Build history of the part. All positions in model axes, mm. A direction names the side the tool comes from. Coordinates: 2 decimals unless noted, no trailing zeros. Order: outer loops, then holes, each group sorted by start corner. A loop starts at its lowest first (then second) coordinate and runs counter-clockwise, first axis right, second up. Notation, with made-up numbers: (50.25, -31) - (69.25, -31) arc R16 cw to (69.25, -13) - close; hole circle Ø2 at (0.5, -5.75). An arc over 180 degrees is marked (long way). Write each question's results on one line, items separated by ' | '.
from build123d import *

# Parameters (mm, degrees)
BOSS_EXTRUDE1_DEPTH = 30
BOSS_EXTRUDE2_DEPTH = 30
SKETCH5_W           = 20
SKETCH5_H           = 30
CUT_EXTRUDE1_DEPTH  = 71
SKETCH6_W           = 30
SKETCH6_H           = 10
CUT_EXTRUDE2_DEPTH  = 40
CUT_EXTRUDE3_DEPTH  = 71


with BuildPart() as part:
    # Sketch1 → Boss-Extrude1 (new body)
    with BuildSketch(Plane(origin=(0, 0, 0), x_dir=(1, 0, 0), z_dir=(0, 1, 0))):
        Polygon((0, 0), (90, 0), (90, -70), (60, -70), (60, -60), (50, -60), (10, -40), (10, -30), (0, -30), align=None)
    extrude(amount=BOSS_EXTRUDE1_DEPTH)

    # Sketch3 → Boss-Extrude2 (add)
    with BuildSketch(Plane(origin=(0, 30, 0), x_dir=(1, 0, 0), z_dir=(0, 1, 0))):
        Polygon((0, 0), (90, 0), (90, -70), (60, -70), (60, -30), (0, -30), align=None)
    extrude(amount=BOSS_EXTRUDE2_DEPTH)

    # Sketch5 → Cut-Extrude1 (cut, through all)
    with BuildSketch(Plane.XY.offset(70)):
        with Locations((80, 25)):
            Rectangle(SKETCH5_W, SKETCH5_H)
    extrude(amount=-CUT_EXTRUDE1_DEPTH, mode=Mode.SUBTRACT)

    # Sketch6 → Cut-Extrude2 (cut)
    with BuildSketch(Plane.XY.offset(70)):
        with Locations((75, 55)):
            Rectangle(SKETCH6_W, SKETCH6_H)
    extrude(amount=-CUT_EXTRUDE2_DEPTH, mode=Mode.SUBTRACT)

    # Sketch7 → Cut-Extrude3 (cut, through all)
    with BuildSketch(Plane(origin=(0, 0, 0), x_dir=(-1, 0, 0), z_dir=(0, 0, -1))):
        Polygon((-40, 60), (-40, 50), (-20, 40), (0, 40), (0, 60), align=None)
    extrude(amount=-CUT_EXTRUDE3_DEPTH, mode=Mode.SUBTRACT)


solid = part.part
1. Band-saw the part on A-A on x = 81. Give the cut face in (y, z).
Solved:
outline: (0, 0) - (10, 0) - (10, 70) - (0, 70) - close; (40, 0) - (60, 0) - (60, 30) - (50, 30) - (50, 70) - (40, 70) - close
2. Band-saw the part on D-D on x = 25.5. Give the cut face in (y, z), then the cut area to 4 significant figures.
Solved:
outline: (0, 0) - (42.75, 0) - (42.75, 30) - (30, 30) - (30, 47.75) - (0, 47.75) - close | area: 1,815 mm2
3. Probe line 1 (Y direction, x = 70.5, z = 34); line 2 (X direction, y = 17, z = 16.5); line 3 (Y direction, x = 75, z = 26). List the from-to ranges inside material, lowest first.
Solved:
line 1: y = 0 to 10, 40 to 50 | line 2: x = 0 to 70 | line 3: y = 0 to 10, 40 to 60
4. Band-saw the part on B-B on z = 50.5. Give the cut face in (x, y), then the cut area to 3 significant figures.
Solved:
outline: (31, 0) - (90, 0) - (90, 10) - (70, 10) - (70, 40) - (90, 40) - (90, 50) - (60, 50) - (60, 30) - (31, 30) - close | area: 1,770 mm2
5. Tool access for faces 1 (the face through (10, 40, 15)), 2 (the face through (41, 30, 41)), 3 (the face through (80, 40, 35)), 4 (the face through (75, 50, 50)), 5 (the face through (10, 15, 35)): list every direction of +Z, -Z, +X, -X, +Y, -Y with a clear straight run to the whole face (end or side of a thin tool).
Solved:
face 1: +Z, -Z, -X, +Y | face 2: +Z, -X, +Y | face 3: +Z, -Z, +X | face 4: +Z, +X, -X, +Y | face 5: +Z, -X, +Y, -Y
6. Two-plate mould, pull along Y, no slides. Class faces 6 (the face through (80, 10, 35)), 7 (the face through (65, 60, 15)), 8 (the face through (44, 30, 0)), 9 (the face through (56, 0, 27)): +Y half, -Y half, draft (parallel to the pull), parting line (faces both ways), or undercut.
Solved:
face 6: undercut | face 7: +Y half | face 8: draft | face 9: -Y half
7. Drop flat-ended pins along their axis: pin 1 Ø10 at (y, z) = (53.5, 19.5) entering from -X; pin 2 Ø1 at (x, y) = (50, 32) entering from +Z; pin 3 Ø11 at (y, z) = (56.5, 8.5) entering from -X. Give the stop position or say it passes through.
Solved:
pin 1: stops at x = 37 | pin 2: stops at z = 30 | pin 3: stops at x = 40
8. Band-saw the part on C-C on y = 47. Give the cut face in (x, z).
Solved:
outline: (34, 0) - (90, 0) - (90, 70) - (60, 70) - (60, 30) - (34, 30) - close
